Source: CAD feature listing. Evaluate the final solid. Frame: model axes, mm. Face numbers are marked on the shaded views. A direction names the side the tool comes from. Coordinates: 2 decimals unless noted, no trailing zeros. Loops run counter-clockwise (first coordinate to the right, second up) from the corner with the lowest first, then second, coordinate; pieces in that order, holes last.
from build123d import *

# Parameters (mm, degrees)
SKETCH_1_W          = 4
SKETCH_1_H          = 8
SKETCH_1_R          = 1.95
EXTRUDE_1_DEPTH     = 2
SKETCH_3_R          = 6
CUT_EXTRUDE_1_DEPTH = 10.16515139
SKETCH_2_R          = 1.95
EXTRUDE_3_DEPTH     = 15
FILLET_3_R          = 0.5


with BuildPart() as part:
    # 草图1 → 凸台-拉伸1 (new body)
    with BuildSketch(Plane(origin=(0, 0, 0), x_dir=(1, 0, 0), z_dir=(0, 1, 0))):
        with Locations((2, 4)):
            Rectangle(SKETCH_1_W, SKETCH_1_H)
        with Locations(Location((2, 4, 0), (0, 0, 270))):
            Circle(SKETCH_1_R, mode=Mode.SUBTRACT)
    extrude(amount=EXTRUDE_1_DEPTH)

    # 草图3 → 切除-拉伸1 (cut, through all)
    with BuildSketch(Plane.ZY):
        with Locations((-4, 7)):
            Circle(SKETCH_3_R)
    extrude(amount=-CUT_EXTRUDE_1_DEPTH, mode=Mode.SUBTRACT)

    # 草图2 → 凸台-拉伸3 (add)
    with BuildSketch(Plane.XZ):
        with Locations(Location((2, -4, 0), (0, 0, 270))):
            Circle(SKETCH_2_R)
    extrude(amount=-EXTRUDE_3_DEPTH)

    # 圆角3
    fillet_3_edges = [part.edges().sort_by_distance(p)[0] for p in [
        (4, 2, -0.341687605),
        (2, 2, -8),
        (4, 2, -7.658312395),
        (0, 2, -0.341687605),
        (2, 2, -0.68337521),
        (2, 2, -7.31662479),
        (2, 15, -2.05),
        (0, 2, -7.658312395),
        (2, 0, -8),
        (4, 0, -4),
        (2, 0, 0),
        (0, 0, -4),
        (2, 2, 0),
    ]]
    fillet(fillet_3_edges, radius=FILLET_3_R)


solid = part.part
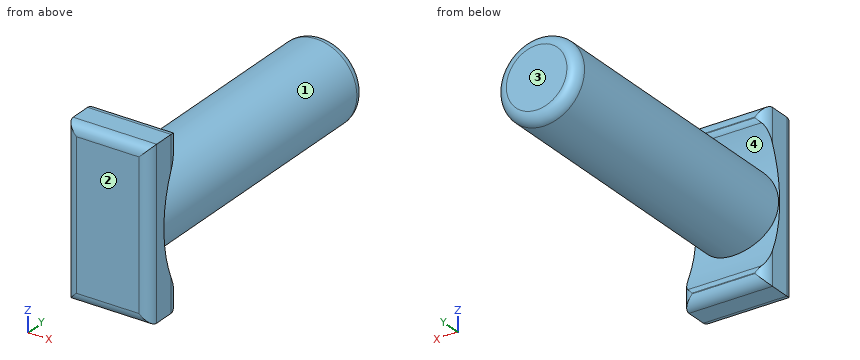
Q1. Section C-C, the plane y = 6.75. Return the cut outline in (x, z), plus the area to 3 significant figures.
Q2. Line query: line 1 along Z through (x, y) = (3.35, 1.75); line 2 along Z through (x, y) = (2, 9.5); line 3 along X through (y, z) = (9.5, -4.75). Output: solid intervals per line, ascending.
Q3. Section A-A, the plane z = -4. Return the cut outline in (x, y).
Q4. Contact query for a flat-ended pin moving along its axis: pin 1 Ø1.5 at (x, y) = (3, 8.5) entering from -Z. Output: stop coordinate, or through.
Q5. Section D-D, the plane z = -6.75. Return the cut outline in (x, y).
Q6. Access query for the marked faces 1 and 2. Directions: +Z, -Z, +X, -X, +Y, -Y. A direction counts if a zero-diameter tool reaches every point of the face in a straight line with its end or side. Return the directions, or none.
Q7. Draft query along Z for the marked faces 3 and 4. Return one class per face: +Z half, -Z half, draft (parallel to the pull), parting line (faces both ways), or undercut.
Derived:
1. outline: circle Ø3.9 at (2, -4)
1. area: 11.9 mm2
2. line 1: z = -7.93 to -6.9, -5.41 to -2.59, -1.1 to -0.07
2. line 2: z = -5.95 to -2.05
2. line 3: x = 0.2 to 3.8
3. outline: (0, 0.5) arc R0.5 ccw to (0.5, 0) - (3.5, 0) arc R0.5 ccw to (4, 0.5) - (4, 1) - (3.95, 1) - (3.95, 14.5) arc R0.5 ccw to (3.45, 15) - (0.55, 15) arc R0.5 ccw to (0.05, 14.5) - (0.05, 1) - (0, 1) - close
4. pin 1: stops at z = -5.93
5. outline: (0, 0.5) arc R0.5 ccw to (0.5, 0) - (3.5, 0) arc R0.5 ccw to (4, 0.5) - (4, 1.5) arc R0.5 ccw to (3.97, 1.67) - (0.03, 1.67) arc R0.5 ccw to (0, 1.5) - close
6. face 1: +Y
6. face 2: +Z, -Z, +X, -X, -Y
7. face 3: draft
7. face 4: undercut
